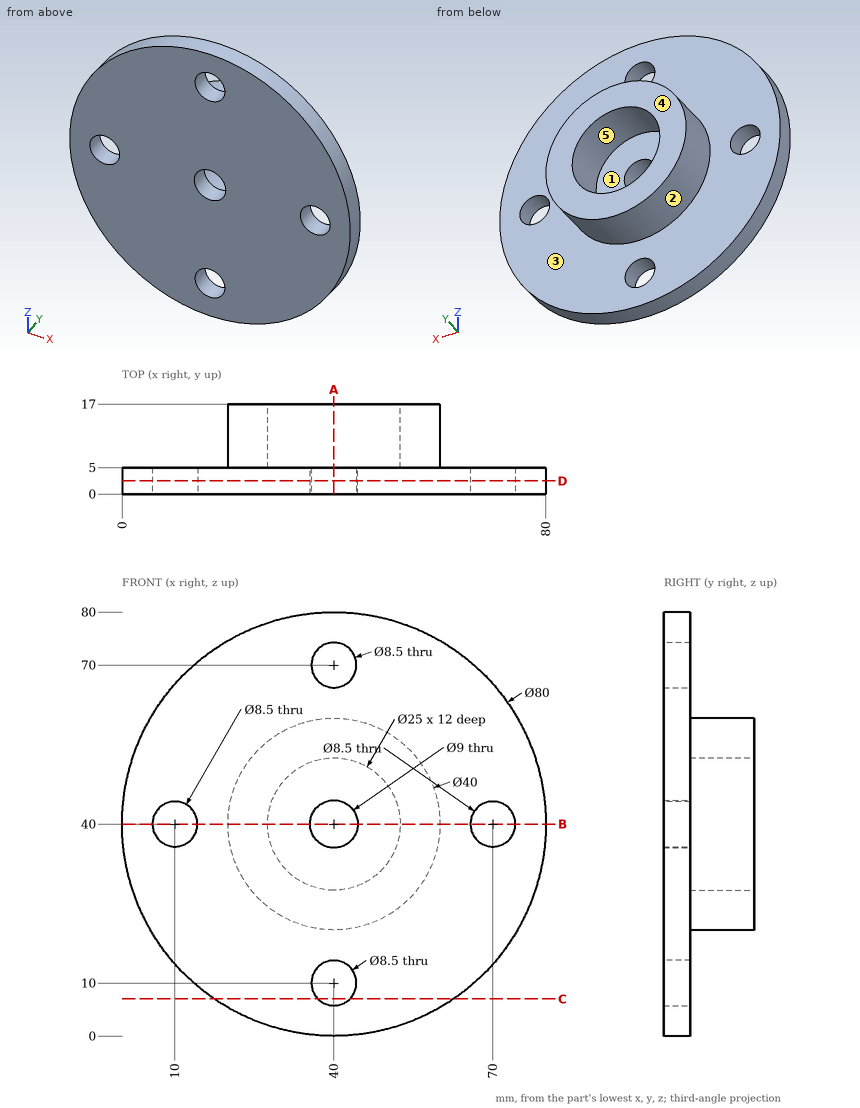
Design review of the part shown in the three views and the two pictorial views. Dimensions are in mm from the part's minimum x, y and z. A direction names the side the tool comes from. Round coordinates to 2 decimals unless told otherwise and drop trailing zeros. Order: outer loops, then holes, each group sorted by start corner. A loop starts at its lowest first (then second) coordinate and runs counter-clockwise, first axis right, second up. Notation, with made-up numbers: (17, 26) -> (67, 26) arc R18 cw to (67, 53) -> close; hole circle Ø10 at (9.25, 48.25). An arc over 180 degrees is marked (long way). Write item = value, one per line. Start each with the question number.
1) Insertion check: pin 1 (4 mm diameter, centred on y = 14.5, z = 55, fed in from -X); pin 2 (1 mm diameter, centred on x = 8, y = 3, fed in from +Z); pin 3 (11 mm diameter, centred on x = 40, z = 70, fed in from +Y); pin 4 (1.5 mm diameter, centred on x = 71.5, z = 39, fed in from +Y). Each pin has a flat end and moves straight along its axis. Give the tip position at first contact, or say it passes through.
2) Take a section at D-D on y = 2.5. State the section outline as (x, z) points.
3) Tool access review of the marked faces 4 and 5: name each direction out of +Z, -Z, +X, -X, +Y, -Y from which nothing blocks a thin tool from reaching the whole face with its end or side.
4) Take a section at C-C on z = 7. State the section outline as (x, y) points.
5) Take a section at A-A on x = 40. State the section outline as (y, z) points, plus the area to 3 significant figures.
6) Take a section at B-B on z = 40. State the section outline as (x, y) points, plus the area to 3 significant figures.
7) The part is to be moulded in two halves that separate along Z. For the marked faces 1, 2 and 3, say which applies: +Z half, -Z half, draft (parallel to the pull), parting line (faces both ways), or undercut.
8) To check wall thickness, follow line 1 (X direction, y = 2, z = 40); line 2 (X direction, y = 9.25, z = 40); line 3 (Z direction, x = 40.5, y = 13.5). State the ranges of each line that lie inside material, in increasing order. Write a range as from..to.
Verdict:
q1.pin_1 = 24.8
q1.pin_2 = 64.65
q1.pin_3 = 5
q1.pin_4 = through
q2.outline = circle Ø80 at (40, 40); hole circle Ø8.5 at (10, 40); hole circle Ø9 at (40, 40); hole circle Ø8.5 at (40, 10); hole circle Ø8.5 at (40, 70); hole circle Ø8.5 at (70, 40)
q3.face_4 = +Z, -Z, +X, -X, +Y
q3.face_5 = +Y
q4.outline = (17.39, 0) -> (36.99, 0) -> (36.99, 5) -> (17.39, 5) -> close; (43.01, 0) -> (62.61, 0) -> (62.61, 5) -> (43.01, 5) -> close
q5.outline = (0, 0) -> (5, 0) -> (5, 5.75) -> (0, 5.75) -> close; (0, 14.25) -> (5, 14.25) -> (5, 20) -> (17, 20) -> (17, 27.5) -> (5, 27.5) -> (5, 35.5) -> (0, 35.5) -> close; (0, 44.5) -> (5, 44.5) -> (5, 52.5) -> (17, 52.5) -> (17, 60) -> (5, 60) -> (5, 65.75) -> (0, 65.75) -> close; (0, 74.25) -> (5, 74.25) -> (5, 80) -> (0, 80) -> close
q5.area = 450 mm2
q6.outline = (0, 0) -> (5.75, 0) -> (5.75, 5) -> (0, 5) -> close; (14.25, 0) -> (35.5, 0) -> (35.5, 5) -> (27.5, 5) -> (27.5, 17) -> (20, 17) -> (20, 5) -> (14.25, 5) -> close; (44.5, 0) -> (65.75, 0) -> (65.75, 5) -> (60, 5) -> (60, 17) -> (52.5, 17) -> (52.5, 5) -> (44.5, 5) -> close; (74.25, 0) -> (80, 0) -> (80, 5) -> (74.25, 5) -> close
q6.area = 450 mm2
q7.face_1 = undercut
q7.face_2 = parting line
q7.face_3 = draft
q8.line_1 = 0..5.75, 14.25..35.5, 44.5..65.75, 74.25..80
q8.line_2 = 20..27.5, 52.5..60
q8.line_3 = 20.01..27.51, 52.49..59.99
